```python
from build123d import *

# Parameters (mm, degrees)
BOSS_EXTRUDE1_DEPTH = 1.2
SKETCH4_W           = 62.7
SKETCH4_H           = 158
BOSS_EXTRUDE3_DEPTH = 3.2
SKETCH6_W           = 13.5
SKETCH6_H           = 11.65
SKETCH6_R           = 1.1
SKETCH6_H_2         = 29.2
BOSS_EXTRUDE4_DEPTH = 5.1
SKETCH7_W           = 0.1
SKETCH7_H           = 11.65
SKETCH7_H_2         = 29.2
BOSS_EXTRUDE5_DEPTH = 3.2
CUT_EXTRUDE5_DEPTH  = 5.1
CUT_EXTRUDE6_DEPTH  = 5.2
SKETCH11_R          = 1.2
CUT_EXTRUDE7_DEPTH  = 5.4
CUT_EXTRUDE8_DEPTH  = 5
BOSS_EXTRUDE6_DEPTH = 5
CUT_EXTRUDE9_DEPTH  = 5
BOSS_EXTRUDE7_START = 5
BOSS_EXTRUDE7_DEPTH = 5
SKETCH20_W          = 8
SKETCH20_H          = 7.2
CUT_EXTRUDE10_DEPTH = 3.6
CUT_EXTRUDE12_DEPTH = 1.8
CUT_EXTRUDE13_START = -5.4
SKETCH23_R          = 1.2
CUT_EXTRUDE13_DEPTH = 5.4
SKETCH24_R          = 0.9
CUT_EXTRUDE14_DEPTH = 96.780634786
CHAMFER1_SIZE       = 1.1
SKETCH26_R          = 2
CUT_EXTRUDE15_DEPTH = 12
CUT_EXTRUDE16_START = 12
SKETCH27_R          = 2
CUT_EXTRUDE16_DEPTH = 12
CUT_EXTRUDE17_START = -3.6
CUT_EXTRUDE17_DEPTH = 1.8
CUT_EXTRUDE18_REACH = 97.781
SKETCH29_W          = 6.8
SKETCH29_H          = 6.1
CUT_EXTRUDE19_DEPTH = 3.2
CUT_EXTRUDE20_REACH = 97.781
SKETCH32_R          = 1.1
CHAMFER2_SIZE       = 0.9


with BuildPart() as part:
    # Sketch1 → Boss-Extrude1 (new body)
    with BuildSketch(Plane(origin=(0, 0, 0), x_dir=(1, 0, 0), z_dir=(0, 1, 0))):
        with BuildLine():
            Line((40, 86.8), (-34, 86.8))
            ThreePointArc((-34, 86.8), (-37.323401872, 85.423401872), (-38.7, 82.1))
            Line((-38.7, 82.1), (-38.7, -82.1))
            ThreePointArc((-38.7, -82.1), (-37.323401872, -85.423401872), (-34, -86.8))
            Line((-34, -86.8), (40, -86.8))
            Line((40, -86.8), (40, 86.8))
        make_face()
    extrude(amount=-BOSS_EXTRUDE1_DEPTH)

    # Sketch4 → Boss-Extrude3 (add)
    with BuildSketch(Plane(origin=(0, -1.2, 0), x_dir=(-1, 0, 0), z_dir=(0, -1, 0))):
        with Locations((-8.65, 2.2)):
            Rectangle(SKETCH4_W, SKETCH4_H)
    extrude(amount=BOSS_EXTRUDE3_DEPTH)

    # Sketch6 → Boss-Extrude4 (add)
    # profile 1 of 2: a face of its own
    with BuildSketch(Plane.XZ.offset(1.2)):
        with Locations((-29.55, -70.575)):
            Rectangle(SKETCH6_W, SKETCH6_H)
        with Locations(Location((-25.5, -68.35, 0), (0, 0, 270))):
            Circle(SKETCH6_R, mode=Mode.SUBTRACT)
    # profile 2 of 2: a face of its own
    with BuildSketch(Plane.XZ.offset(1.2)):
        with Locations((-29.55, 56.05)):
            Rectangle(SKETCH6_W, SKETCH6_H_2)
        with Locations(Location((-25.5, 56.05, 0), (0, 0, 270))):
            Circle(SKETCH6_R, mode=Mode.SUBTRACT)
    extrude(amount=BOSS_EXTRUDE4_DEPTH)

    # Sketch7 → Boss-Extrude5 (add)
    with BuildSketch(Plane.XZ.offset(1.2)):
        with Locations((-22.75, -70.575)):
            Rectangle(SKETCH7_W, SKETCH7_H)
        with Locations((-22.75, 56.05)):
            Rectangle(SKETCH7_W, SKETCH7_H_2)
    extrude(amount=BOSS_EXTRUDE5_DEPTH)

    # Sketch10 → Cut-Extrude5 (cut)
    with BuildSketch(Plane.XZ.offset(6.3)):
        Polygon((-25.959839262, 43.33044604), (-25.695559806, 41.45), (-39.339908081, 41.45), align=None)
        Polygon((-29.578339887, 69.077415827), (-29.79935218, 70.65), (-36.3, 70.65), (-36.3, 68.132748105), align=None)
    extrude(amount=-CUT_EXTRUDE5_DEPTH, mode=Mode.SUBTRACT)

    # Sketch9 → Cut-Extrude6 (cut)
    with BuildSketch(Plane(origin=(0, 0, 0), x_dir=(1, 0, 0), z_dir=(0, 1, 0))):
        Polygon((-34.925787458, -68.325881082), (-34.229921954, -63.374540738), (-28.882474382, -64.126075484), (-29.578339887, -69.077415827), align=None)
        Polygon((-25.959839262, -43.33044604), (-31.307286833, -42.578911295), (-32.003152338, -47.530251639), (-26.655704767, -48.281786384), align=None)
    extrude(amount=-CUT_EXTRUDE6_DEPTH, mode=Mode.SUBTRACT)

    # Sketch11 → Cut-Extrude7 (cut)
    with BuildSketch(Plane(origin=(-9.39719998, 0, 66.864552213), x_dir=(0.9902680687415714, 0, 0.13917310096005855), z_dir=(-0.13917310096005855, 0, 0.9902680687415714))):
        with Locations((-22.37676735, -2.5)):
            Circle(SKETCH11_R)
    extrude(amount=-CUT_EXTRUDE7_DEPTH, mode=Mode.SUBTRACT)

    # Sketch15 → Cut-Extrude8 (cut)
    with BuildSketch(Plane(origin=(-9.39719998, 0, 66.864552213), x_dir=(0.9902680687415714, 0, 0.13917310096005855), z_dir=(-0.13917310096005855, 0, 0.9902680687415714))):
        Polygon((-25.902439291, 0), (-25.07676735, 0), (-25.07676735, -2.879460254), align=None)
    extrude(amount=CUT_EXTRUDE8_DEPTH, mode=Mode.SUBTRACT)

    # Sketch17 → Boss-Extrude6 (add)
    with BuildSketch(Plane(origin=(-9.39719998, 0, 66.864552213), x_dir=(0.9902680687415714, 0, 0.13917310096005855), z_dir=(-0.13917310096005855, 0, 0.9902680687415714))):
        with BuildLine():
            Line((-25.07676735, -2.879460254), (-24.972173929, -3.244220861))
            ThreePointArc((-24.972173929, -3.244220861), (-22.000999977, -5.173723786), (-19.67676735, -2.5))
            Line((-19.67676735, -2.5), (-19.67676735, -6.3))
            Line((-19.67676735, -6.3), (-25.07676735, -6.3))
            Line((-25.07676735, -6.3), (-25.07676735, -2.879460254))
        make_face()
    extrude(amount=BOSS_EXTRUDE6_DEPTH)

    # Sketch18 → Cut-Extrude9 (cut)
    with BuildSketch(Plane(origin=(-7.170430365, 0, 51.020263113), x_dir=(-0.9902680687415715, 0, -0.13917310096005736), z_dir=(0.13917310096005736, 0, -0.9902680687415715))):
        Polygon((25.902439291, 0), (25.07676735, 0), (25.07676735, -2.879460254), align=None)
    extrude(amount=CUT_EXTRUDE9_DEPTH, mode=Mode.SUBTRACT)

    # Sketch19 → Boss-Extrude7 (add)
    with BuildSketch(Plane(origin=(-7.170430365, 0, 51.020263113), x_dir=(-0.9902680687415715, 0, -0.13917310096005736), z_dir=(0.13917310096005736, 0, -0.9902680687415715)).offset(BOSS_EXTRUDE7_START)):
        with BuildLine():
            Line((25.07676735, -2.879460254), (24.972173929, -3.244220861))
            ThreePointArc((24.972173929, -3.244220861), (22.000999977, -5.173723786), (19.67676735, -2.5))
            Line((19.67676735, -2.5), (19.67676735, -6.3))
            Line((19.67676735, -6.3), (25.07676735, -6.3))
            Line((25.07676735, -6.3), (25.07676735, -2.879460254))
        make_face()
    extrude(amount=-BOSS_EXTRUDE7_DEPTH)

    # Sketch20 → Cut-Extrude10 (cut)
    with BuildSketch(Plane.XZ.offset(6.3)):
        with Locations((-32.3, 56.05)):
            Rectangle(SKETCH20_W, SKETCH20_H)
    extrude(amount=-CUT_EXTRUDE10_DEPTH, mode=Mode.SUBTRACT)

    # Sketch22 → Cut-Extrude12 (cut)
    with BuildSketch(Plane(origin=(0, -2.7, 0), x_dir=(-1, 0, 0), z_dir=(0, -1, 0))):
        Polygon((24.056624327, -58.55), (26.943375673, -58.55), (28.3, -58.55), (28.3, -53.55), (26.943375673, -53.55), (24.056624327, -53.55), (22.613248654, -56.05), align=None)
    extrude(amount=CUT_EXTRUDE12_DEPTH, mode=Mode.SUBTRACT)

    # Sketch23 → Cut-Extrude13 (cut)
    with BuildSketch(Plane(origin=(-7.170430365, 0, 51.020263113), x_dir=(-0.9902680687415715, 0, -0.13917310096005736), z_dir=(0.13917310096005736, 0, -0.9902680687415715)).offset(CUT_EXTRUDE13_START)):
        with Locations(Location((22.37676735, -2.5, 0), (0, 0, 180))):
            Circle(SKETCH23_R)
    extrude(amount=CUT_EXTRUDE13_DEPTH, mode=Mode.SUBTRACT)

    # Sketch24 → Cut-Extrude14 (cut, through all)
    with BuildSketch(Plane(origin=(0, 0, 0), x_dir=(1, 0, 0), z_dir=(0, 1, 0))):
        with Locations(Location((-32.30933316, -49.70884139, 0), (0, 0, 270))):
            Circle(SKETCH24_R)
        with Locations(Location((-26.961885589, -50.460376135, 0), (0, 0, 270))):
            Circle(SKETCH24_R)
        with Locations(Location((-28.57629356, -61.947485732, 0), (0, 0, 270))):
            Circle(SKETCH24_R)
        with Locations(Location((-33.923741132, -61.195950987, 0), (0, 0, 270))):
            Circle(SKETCH24_R)
    extrude(amount=-CUT_EXTRUDE14_DEPTH, mode=Mode.SUBTRACT)

    # Chamfer1
    chamfer1_edges = [part.edges().sort_by_distance(p)[0] for p in [
        (-32.30933316, 0, 48.80884139),
        (-33.923741132, 0, 60.295950987),
        (-28.57629356, 0, 61.047485732),
        (-26.961885589, 0, 49.560376135),
    ]]
    chamfer(chamfer1_edges, length=CHAMFER1_SIZE)

    # Sketch26 → Cut-Extrude15 (cut)
    with BuildSketch(Plane(origin=(-6.47456486, 0, 46.068922769), x_dir=(-0.9902680687415714, 0, -0.13917310096005867), z_dir=(0.13917310096005867, 0, -0.9902680687415714))):
        with Locations((22.37676735, -2.5)):
            Circle(SKETCH26_R)
    extrude(amount=CUT_EXTRUDE15_DEPTH, mode=Mode.SUBTRACT)

    # Sketch27 → Cut-Extrude16 (cut)
    with BuildSketch(Plane(origin=(-10.093065485, 0, 71.815892556), x_dir=(0.9902680687415714, 0, 0.1391731009600588), z_dir=(-0.1391731009600588, 0, 0.9902680687415714)).offset(CUT_EXTRUDE16_START)):
        with Locations((-22.37676735, -2.5)):
            Circle(SKETCH27_R)
    extrude(amount=-CUT_EXTRUDE16_DEPTH, mode=Mode.SUBTRACT)

    # Sketch28 → Cut-Extrude17 (cut)
    with BuildSketch(Plane.XZ.offset(6.3).offset(CUT_EXTRUDE17_START)):
        Polygon((-26.943375673, -70.85), (-24.056624327, -70.85), (-22.613248654, -68.35), (-24.056624327, -65.85), (-26.943375673, -65.85), (-28.386751346, -65.85), (-28.386751346, -64.75), (-35.186751346, -64.75), (-35.186751346, -70.85), align=None)
    extrude(amount=CUT_EXTRUDE17_DEPTH, mode=Mode.SUBTRACT)

    # Sketch29 → Cut-Extrude18 (cut, up to next)
    with BuildSketch(Plane.XZ.offset(6.3), mode=Mode.PRIVATE) as cut_extrude18_sk1:
        with Locations((-31.786751346, -67.8)):
            Rectangle(SKETCH29_W, SKETCH29_H)
    cut_extrude18_tool1 = extrude(cut_extrude18_sk1.sketch, amount=-CUT_EXTRUDE18_REACH, mode=Mode.PRIVATE) & part.part
    add(cut_extrude18_tool1.solids().sort_by_distance((-31.786751, -6.3, -67.8))[0], mode=Mode.SUBTRACT)

    # Sketch31 → Cut-Extrude19 (cut)
    with BuildSketch(Plane.XZ.offset(4.4)):
        Polygon((40, 70), (32.8, 62.8), (32.8, -62.8), (40, -70), align=None)
    extrude(amount=-CUT_EXTRUDE19_DEPTH, mode=Mode.SUBTRACT)

    # Sketch32 → Cut-Extrude20 (cut, up to next)
    with BuildSketch(Plane(origin=(0, 0, 0), x_dir=(1, 0, 0), z_dir=(0, 1, 0)), mode=Mode.PRIVATE) as cut_extrude20_sk1:
        with Locations(Location((36.4, 50, 0), (0, 0, 270))):
            Circle(SKETCH32_R)
    cut_extrude20_tool1 = extrude(cut_extrude20_sk1.sketch, amount=-CUT_EXTRUDE20_REACH, mode=Mode.PRIVATE) & part.part
    # Sketch32 → Cut-Extrude20 (cut, up to next)
    with BuildSketch(Plane(origin=(0, 0, 0), x_dir=(1, 0, 0), z_dir=(0, 1, 0)), mode=Mode.PRIVATE) as cut_extrude20_sk2:
        with Locations(Location((36.4, 0, 0), (0, 0, 270))):
            Circle(SKETCH32_R)
    cut_extrude20_tool2 = extrude(cut_extrude20_sk2.sketch, amount=-CUT_EXTRUDE20_REACH, mode=Mode.PRIVATE) & part.part
    # Sketch32 → Cut-Extrude20 (cut, up to next)
    with BuildSketch(Plane(origin=(0, 0, 0), x_dir=(1, 0, 0), z_dir=(0, 1, 0)), mode=Mode.PRIVATE) as cut_extrude20_sk3:
        with Locations(Location((36.4, -50, 0), (0, 0, 270))):
            Circle(SKETCH32_R)
    cut_extrude20_tool3 = extrude(cut_extrude20_sk3.sketch, amount=-CUT_EXTRUDE20_REACH, mode=Mode.PRIVATE) & part.part
    add(cut_extrude20_tool1.solids().sort_by_distance((36.4, 0, -50))[0], mode=Mode.SUBTRACT)
    add(cut_extrude20_tool2.solids().sort_by_distance((36.4, 0, 0))[0], mode=Mode.SUBTRACT)
    add(cut_extrude20_tool3.solids().sort_by_distance((36.4, 0, 50))[0], mode=Mode.SUBTRACT)

    # Chamfer2
    chamfer2_edges = [part.edges().sort_by_distance(p)[0] for p in [
        (36.4, 0, -51.1),
        (36.4, 0, -1.1),
        (36.4, 0, 48.9),
    ]]
    chamfer(chamfer2_edges, length=CHAMFER2_SIZE)


solid = part.part
```
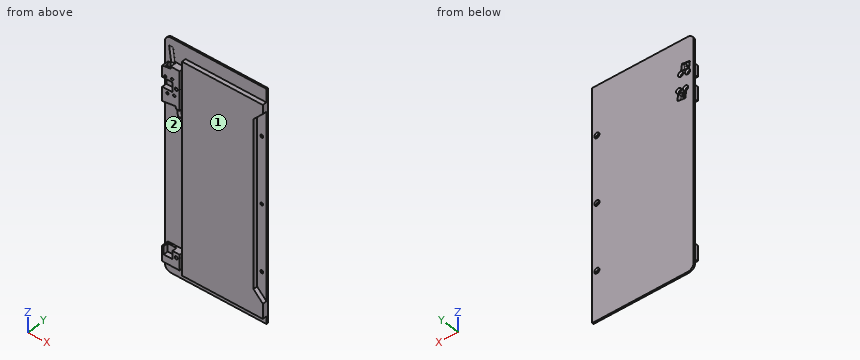
Geometry check sheet. Reference: the model listing, model coordinates, mm. Face numbers are marked on the shaded views. Coordinates: 2 decimals unless noted, no trailing zeros. Order: outer loops, then holes, each group sorted by start corner. A loop starts at its lowest first (then second) coordinate and runs counter-clockwise, first axis right, second up.
Item 1: Scan lines: line 1 along Z through (x, y) = (-25.5, -1.7); line 2 along Z through (x, y) = (-30, -5.25); line 3 along Z through (x, y) = (-25.5, -3). Record each from-to range of solid material in increasing order.
Item 2: Depth check by flat-ended pin: pin 1 (2 mm diameter, centred on y = -5, z = 68.5, fed in from -X); pin 2 (1.5 mm diameter, centred on y = -2.5, z = -5.5, fed in from +X); pin 3 (6 mm diameter, centred on x = 21.5, z = -29.5, fed in from -Y). Enter the tip coordinate at first touch or a pass-through.
Item 3: Section check B-B (x = -0.5). Enter the section's corners in (y, z), plus the area to 3 significant figures.
Item 4: Mould release check, pull along Z, two halves, no side actions. Record for the marked faces 1 and 2: released by +Z, released by -Z, zero draft, split by the parting line, or undercut.
Item 5: Section check A-A (z = -19.5). Enter the section's corners in (x, y), plus the area to 3 significant figures.
Check sheet entries:
1. line 1: z = -76.4 to -69.45, -67.25 to -64.75, 41.45 to 54.95, 57.15 to 70.65
1. line 2: z = -76.4 to -70.85, 42.76 to 52.45, 59.65 to 69.02
1. line 3: z = -76.4 to -70.85, -65.85 to -64.75, 41.45 to 53.55, 58.55 to 70.65
2. pin 1: stops at x = -36.3
2. pin 2: stops at x = 32.8
2. pin 3: stops at y = -4.4
3. outline: (-4.4, -81.2) - (-1.2, -81.2) - (-1.2, -86.8) - (0, -86.8) - (0, 86.8) - (-1.2, 86.8) - (-1.2, 76.8) - (-4.4, 76.8) - close
3. area: 714 mm2
4. face 1: zero draft
4. face 2: undercut
5. outline: (-38.7, -1.2) - (-22.7, -1.2) - (-22.7, -4.4) - (32.8, -4.4) - (32.8, -1.2) - (40, -1.2) - (40, 0) - (-38.7, 0) - close
5. area: 272 mm2
